Part model, mm, in its own coordinate system. Round coordinates to 2 decimals unless told otherwise and drop trailing zeros. Order: outer loops, then holes, each group sorted by start corner. A loop starts at its lowest first (then second) coordinate and runs counter-clockwise, first axis right, second up. Notation, with made-up numbers: (19.25, -6.75) -> (74.25, -6.75) arc R29 cw to (74.25, 24.25) -> close; hole circle Ø10 at (6.25, -23). An arc over 180 degrees is marked (long way). Use CSV: the item, a comma, the result in double quotes.
```python
from build123d import *

# Parameters (mm, degrees)
SKETCH1_W           = 600
SKETCH1_H           = 300
BOSS_EXTRUDE1_DEPTH = 3
SKETCH2_W           = 30
SKETCH2_H           = 3
SKETCH2_W_2         = 3
SKETCH2_H_2         = 30
CUT_EXTRUDE1_DEPTH  = 5
SKETCH3_W           = 3
SKETCH3_H           = 30
CUT_EXTRUDE2_DEPTH  = 10
SKETCH4_W           = 3
SKETCH4_H           = 30
CUT_EXTRUDE3_DEPTH  = 5


with BuildPart() as part:
    # Sketch1 → Boss-Extrude1 (new body)
    with BuildSketch(Plane(origin=(0, 0, 0), x_dir=(1, 0, 0), z_dir=(0, 1, 0))):
        with Locations((300, 150)):
            Rectangle(SKETCH1_W, SKETCH1_H)
    extrude(amount=BOSS_EXTRUDE1_DEPTH)

    # Sketch2 → Cut-Extrude1 (cut)
    with BuildSketch(Plane(origin=(0, 3, 0), x_dir=(1, 0, 0), z_dir=(0, 1, 0))):
        with Locations((90, 1.5)):
            Rectangle(SKETCH2_W, SKETCH2_H)
        with Locations((30, 1.5)):
            Rectangle(SKETCH2_W, SKETCH2_H)
        with Locations((150, 1.5)):
            Rectangle(SKETCH2_W, SKETCH2_H)
        with Locations((210, 1.5)):
            Rectangle(SKETCH2_W, SKETCH2_H)
        with Locations((270, 1.5)):
            Rectangle(SKETCH2_W, SKETCH2_H)
        with Locations((330, 1.5)):
            Rectangle(SKETCH2_W, SKETCH2_H)
        with Locations((390, 1.5)):
            Rectangle(SKETCH2_W, SKETCH2_H)
        with Locations((450, 1.5)):
            Rectangle(SKETCH2_W, SKETCH2_H)
        with Locations((510, 1.5)):
            Rectangle(SKETCH2_W, SKETCH2_H)
        with Locations((570, 1.5)):
            Rectangle(SKETCH2_W, SKETCH2_H)
        with Locations((570, 298.5)):
            Rectangle(SKETCH2_W, SKETCH2_H)
        with Locations((510, 298.5)):
            Rectangle(SKETCH2_W, SKETCH2_H)
        with Locations((450, 298.5)):
            Rectangle(SKETCH2_W, SKETCH2_H)
        with Locations((390, 298.5)):
            Rectangle(SKETCH2_W, SKETCH2_H)
        with Locations((330, 298.5)):
            Rectangle(SKETCH2_W, SKETCH2_H)
        with Locations((270, 298.5)):
            Rectangle(SKETCH2_W, SKETCH2_H)
        with Locations((210, 298.5)):
            Rectangle(SKETCH2_W, SKETCH2_H)
        with Locations((150, 298.5)):
            Rectangle(SKETCH2_W, SKETCH2_H)
        with Locations((90, 298.5)):
            Rectangle(SKETCH2_W, SKETCH2_H)
        with Locations((30, 298.5)):
            Rectangle(SKETCH2_W, SKETCH2_H)
        with Locations((1.5, 210)):
            Rectangle(SKETCH2_W_2, SKETCH2_H_2)
        with Locations((1.5, 270)):
            Rectangle(SKETCH2_W_2, SKETCH2_H_2)
        with Locations((1.5, 150)):
            Rectangle(SKETCH2_W_2, SKETCH2_H_2)
        with Locations((1.5, 90)):
            Rectangle(SKETCH2_W_2, SKETCH2_H_2)
        with Locations((1.5, 30)):
            Rectangle(SKETCH2_W_2, SKETCH2_H_2)
        with Locations((598.5, 30)):
            Rectangle(SKETCH2_W_2, SKETCH2_H_2)
        with Locations((598.5, 90)):
            Rectangle(SKETCH2_W_2, SKETCH2_H_2)
        with Locations((598.5, 150)):
            Rectangle(SKETCH2_W_2, SKETCH2_H_2)
        with Locations((598.5, 210)):
            Rectangle(SKETCH2_W_2, SKETCH2_H_2)
        with Locations((598.5, 270)):
            Rectangle(SKETCH2_W_2, SKETCH2_H_2)
    extrude(amount=-CUT_EXTRUDE1_DEPTH, mode=Mode.SUBTRACT)

    # Sketch3 → Cut-Extrude2 (cut)
    with BuildSketch(Plane(origin=(0, 3, 0), x_dir=(1, 0, 0), z_dir=(0, 1, 0))):
        with Locations((68.5, 210)):
            Rectangle(SKETCH3_W, SKETCH3_H)
        with Locations((68.5, 150)):
            Rectangle(SKETCH3_W, SKETCH3_H)
        with Locations((68.5, 90)):
            Rectangle(SKETCH3_W, SKETCH3_H)
        with Locations((161.5, 90)):
            Rectangle(SKETCH3_W, SKETCH3_H)
        with Locations((161.5, 150)):
            Rectangle(SKETCH3_W, SKETCH3_H)
        with Locations((161.5, 210)):
            Rectangle(SKETCH3_W, SKETCH3_H)
        with Locations((438.5, 210)):
            Rectangle(SKETCH3_W, SKETCH3_H)
        with Locations((438.5, 150)):
            Rectangle(SKETCH3_W, SKETCH3_H)
        with Locations((438.5, 90)):
            Rectangle(SKETCH3_W, SKETCH3_H)
        with Locations((531.5, 90)):
            Rectangle(SKETCH3_W, SKETCH3_H)
        with Locations((531.5, 150)):
            Rectangle(SKETCH3_W, SKETCH3_H)
        with Locations((531.5, 210)):
            Rectangle(SKETCH3_W, SKETCH3_H)
    extrude(amount=-CUT_EXTRUDE2_DEPTH, mode=Mode.SUBTRACT)

    # Sketch4 → Cut-Extrude3 (cut)
    with BuildSketch(Plane(origin=(0, 3, 0), x_dir=(1, 0, 0), z_dir=(0, 1, 0))):
        with Locations((215, 180)):
            Rectangle(SKETCH4_W, SKETCH4_H)
        with Locations((215, 120)):
            Rectangle(SKETCH4_W, SKETCH4_H)
        with Locations((385, 120)):
            Rectangle(SKETCH4_W, SKETCH4_H)
        with Locations((385, 180)):
            Rectangle(SKETCH4_W, SKETCH4_H)
    extrude(amount=-CUT_EXTRUDE3_DEPTH, mode=Mode.SUBTRACT)


solid = part.part
```
(1) Cut at C-C, the plane x = 394.5. Give the cut face in (y, z).
Reply:
outline,"(0, -297) -> (3, -297) -> (3, -3) -> (0, -3) -> close"
(2) Cut at B-B, the plane y = 0.55. State how many separate pieces and enclosed holes the cut face has, then the cut area to 3 significant figures.
Reply:
separate pieces,"1"
enclosed holes,"16"
area,"176,000 mm2"
(3) Drop flat-ended pins along their axis: P1, Ø0.9, axis at y = 2, z = -92.5, coming from the +X side; P2, Ø4, axis at x = 245.5, z = -93, coming from the -Y side; P3, Ø0.9, axis at y = 1, z = -208.5, coming from the -X side; P4, Ø0.9, axis at x = 161.5, y = 2, coming from the -Z side. Give the stop position or say it passes through.
Reply:
P1,"x = 597"
P2,"y = 0"
P3,"x = 3"
P4,"z = -297"
(4) Cut at A-A, the plane z = -155. Give the cut face in (x, y).
Reply:
outline,"(3, 0) -> (67, 0) -> (67, 3) -> (3, 3) -> close; (70, 0) -> (160, 0) -> (160, 3) -> (70, 3) -> close; (163, 0) -> (437, 0) -> (437, 3) -> (163, 3) -> close; (440, 0) -> (530, 0) -> (530, 3) -> (440, 3) -> close; (533, 0) -> (597, 0) -> (597, 3) -> (533, 3) -> close"
(5) Probe probe 1 along X at (y, z) = (0.5, -214); probe 2 along X at (y, z) = (2.4, -176.5); probe 3 along Z at (x, y) = (531, 1.6). List the from-to ranges inside material, lowest first. Write a range as [from, to].
Reply:
probe 1,"[3, 67], [70, 160], [163, 437], [440, 530], [533, 597]"
probe 2,"[0, 213.5], [216.5, 383.5], [386.5, 600]"
probe 3,"[-300, -225], [-195, -165], [-135, -105], [-75, 0]"
